Input: part model. Units: mm. Frame: model coordinates. A direction names the side the tool comes from. Coordinates: 2 decimals unless noted, no trailing zeros. Loops run counter-clockwise (first coordinate to the right, second up) from the corner with the lowest first, then second, coordinate; pieces in that order, holes last.
(1) Mould query, pull axis Y, two halves, no side actions, for faces 1 (the face through (92, -13, 9.525)), 2 (the face through (-1, -25.4, -21)), 3 (the face through (-1, -127, 1)). Classes: released by +Y, released by -Y, zero draft, split by the parting line, or undercut.
(2) Line query: L1, parallel to Y at x = 45, z = 0; L2, parallel to X at y = -105.41, z = -45.75; L3, parallel to Y at x = -44, z = 14. Output: solid intervals per line, ascending.
(3) Contact query for flat-ended pins moving along their axis: P1, Ø12, axis at x = -14, y = 26.5, coming from the +Z side; P2, Ø14, axis at y = -103, z = -2.5, coming from the -X side; P3, Ø20.5, axis at x = 91.5, y = -11, coming from the -Z side. Output: stop coordinate, or through.
(4) Section C-C, the plane y = -79.5. Return loops of the section in (x, z), then the cut area to 3 significant figures.
(5) Section B-B, the plane x = -42. Give the number of separate pieces and of enclosed holes in the cut face, then the cut area to 3 significant figures.
(6) Set-up query: faces 4 (the face through (0, -39.878, 76)), 5 (the face through (0, -39.878, -76)), 6 (the face through (0, -105, -34.798)), 7 (the face through (0, -105, 34.798)). Return all of +Z, -Z, +X, -X, +Y, -Y with unobstructed straight access to the full face (end or side cutting, diameter ignored); none if empty.
```python
from build123d import *

# Parameters (mm, degrees)
F0_R      = 101.6
F1_DEPTH  = 19.05
F2_R      = 19.05
F3_DEPTH  = 76.2
F4_R      = 50.8
F4_R_2    = 19.05
F5_DEPTH  = 31.75
F6_R      = 9.525
F7_DEPTH  = 20.828
F8_R      = 12.7
F9_R      = 25.4
F10_DEPTH = 19.05
F11_R     = 19.05
F12_DEPTH = 25.4
F13_DEPTH = 25.4
F15_DEPTH = 27.94
F17_DEPTH = 25.4
F18_SIZE2 = 1.524
F18_SIZE  = 1.524
F20_R     = 6.35
F21_DEPTH = 16.002
F24_DEPTH = 16.002
F26_R     = 6.35
F27_DEPTH = 16.002
F29_R     = 6.35
F30_DEPTH = 16.002


with BuildPart() as f1:
    # F0 (on Front) → F1 (new body)
    with BuildSketch(Plane.XZ):
        Circle(F0_R)
    extrude(amount=F1_DEPTH)

    # F2 (on face) → F3 (join)
    with BuildSketch(Plane.XZ.offset(19.05)):
        Circle(F2_R)
    extrude(amount=F3_DEPTH)

    # F4 (on face) → F5 (join)
    with BuildSketch(Plane.XZ.offset(95.25)):
        Circle(F4_R)
        Circle(F4_R_2, mode=Mode.SUBTRACT)
        Circle(F4_R_2)
    extrude(amount=F5_DEPTH)

    # F6 (on face) → F7 (join)
    with BuildSketch(Plane.XZ.offset(19.05)):
        with Locations((0, 76.2)):
            Circle(F6_R)
        with Locations((0, -76.578163)):
            Circle(F6_R)
    extrude(amount=F7_DEPTH)

    # F8
    f8_edges = [f1.edges().sort_by_distance(p)[0] for p in [
        (-50.8, -127, 0),
    ]]
    fillet(f8_edges, radius=F8_R)

    # F9 (on face) → F10 (join)
    with BuildSketch(Plane(origin=(0, 0, 0), x_dir=(-1, 0, 0), z_dir=(0, 1, 0))):
        Circle(F9_R)
    extrude(amount=F10_DEPTH)

    # F11 (on face) → F12 (join)
    with BuildSketch(Plane(origin=(0, 19.05, 0), x_dir=(-1, 0, 0), z_dir=(0, 1, 0))):
        Circle(F11_R)
    extrude(amount=F12_DEPTH)

    # F0 (on Front) → F13 (join)
    with BuildSketch(Plane.XZ):
        Circle(F0_R)
    extrude(amount=F13_DEPTH)

    # F14 (on face) → F15 (cut)
    with BuildSketch(Plane.XZ.offset(25.4)):
        Polygon((82.55, 9.525), (82.55, 0), (82.55, -9.525), (120.547909, -9.525), (120.547909, 9.525), align=None)
    extrude(amount=-F15_DEPTH, mode=Mode.SUBTRACT)

    # F16 (on face) → F17 (cut)
    with BuildSketch(Plane.XZ.offset(25.4)):
        Polygon((-82.55, -9.525), (-82.55, 0), (-82.55, 9.525), (-117.500194, 9.525), (-117.500194, -9.525), align=None)
    extrude(amount=-F17_DEPTH, mode=Mode.SUBTRACT)

    # F18
    f18_edges = [f1.edges().sort_by_distance(p)[0] for p in [
        (-9.525, -39.878, 76.2),
        (-9.525, -39.878, -76.578163),
    ]]
    chamfer(f18_edges, length=F18_SIZE, length2=F18_SIZE2)

    # F20 (on offset) → F21 (cut)
    with BuildSketch(Plane.XY.offset(50.8)):
        with Locations((0, -105.41)):
            Circle(F20_R)
    extrude(amount=-F21_DEPTH, mode=Mode.SUBTRACT)

    # F23 (on offset) → F24 (cut)
    with BuildSketch(Plane.XY.offset(-50.8)):
        with BuildLine():
            ThreePointArc((0, -99.06), (-4.490128, -109.900128), (6.35, -105.41))
            ThreePointArc((6.35, -105.41), (4.490128, -100.919872), (0, -99.06))
        make_face()
    extrude(amount=F24_DEPTH, mode=Mode.SUBTRACT)

    # F26 (on offset) → F27 (cut)
    with BuildSketch(Plane.YZ.offset(50.8)):
        with Locations((-105.41, 0)):
            Circle(F26_R)
    extrude(amount=-F27_DEPTH, mode=Mode.SUBTRACT)

    # F29 (on offset) → F30 (cut)
    with BuildSketch(Plane.YZ.offset(-50.8)):
        with Locations((-105.41, 0)):
            Circle(F29_R)
    extrude(amount=F30_DEPTH, mode=Mode.SUBTRACT)


solid = f1.part
```
Report:
1. face 1: zero draft
1. face 2: undercut
1. face 3: released by -Y
2. L1: y = -124.96 to -111.76, -99.06 to -95.25, -25.4 to 0
2. L2: x = -22.08 to -6.35, 6.35 to 22.08
2. L3: y = -124.1 to -95.25, -25.4 to 0
3. P1: stops at z = 17.29
3. P2: stops at x = -50.8
3. P3: stops at z = -61
4. outline: circle Ø38.1 at (0, 0)
4. area: 1,140 mm2
5. separate pieces: 2
5. enclosed holes: 1
5. area: 6,230 mm2
6. face 4: +Z, +X, -X, -Y
6. face 5: -Z, +X, -X, -Y
6. face 6: -Z
6. face 7: +Z
